```python
from build123d import *

# Parameters (mm, degrees)
SKETCH1_R               = 7.5
BOSS_EXTRUDE1_DEPTH     = 3
SKETCH3_R               = 2.5
BOSS_EXTRUDE3_DEPTH     = 15
FILLET1_R               = 1
SKETCH4_R               = 12.375
SKETCH4_R_2             = 2.375
CUT_EXTRUDE_THIN1_DEPTH = 0.5


with BuildPart() as part:
    # Sketch1 → Boss-Extrude1 (new body)
    with BuildSketch(Plane.XY):
        Circle(SKETCH1_R)
    extrude(amount=BOSS_EXTRUDE1_DEPTH)

    # Sketch3 → Boss-Extrude3 (add)
    with BuildSketch(Plane.XY.offset(3)):
        Circle(SKETCH3_R)
    extrude(amount=BOSS_EXTRUDE3_DEPTH)

    # Fillet1
    fillet1_edges = [part.edges().sort_by_distance(p)[0] for p in [
        (-7.5, 0, 0),
        (-2.5, 0, 18),
    ]]
    fillet(fillet1_edges, radius=FILLET1_R)

    # Sketch4 → Cut-Extrude-Thin1 (cut)
    with BuildSketch(Plane.XY.offset(15)):
        Circle(SKETCH4_R)
        Circle(SKETCH4_R_2, mode=Mode.SUBTRACT)
    extrude(amount=CUT_EXTRUDE_THIN1_DEPTH, mode=Mode.SUBTRACT)


solid = part.part
```
Model file for the job. Use its own axes, mm. Coordinates: 2 decimals unless noted, no trailing zeros. Loops run counter-clockwise (first coordinate to the right, second up) from the corner with the lowest first, then second, coordinate; pieces in that order, holes last. Notation, with made-up numbers: (-10, 26.5) - (2, 26.5) arc R21 ccw to (2, 52.5) - close; hole circle Ø9 at (19, 74.25). An arc over 180 degrees is marked (long way). Answer as a JSON object with one key per item and string values. Group by question number.
(1) Cut at C-C (z = 15.25). Give the cut face in (x, y) (3 decimals), then the cut area to 3 significant figures.
(2) Flat gauge pins, fed straight in: pin 1 (6 mm diameter, centred on x = 5.5, z = 4, fed in from -Y); pin 2 (8 mm diameter, centred on y = 6, z = 6, fed in from -X). Where does each tip first touch, or does it go through?
(3) Cut at A-A (y = 0). Give the cut face in (x, z) (3 decimals).
(4) Probe line 1 along Z through (x, y) = (-2.75, -4); line 2 along X through (y, z) = (2, 5.5); line 3 along Z through (x, y) = (0, -1.75). List the from-to ranges inside material, lowest first.
(5) Cut at D-D (z = 5.75). Give the cut face in (x, y).
(6) Two-plate mould, pull along Z, no slides. Class faces 1 (the face through (1.096, -2.107, 15.246)), 2 (the face through (0, 0, 18)), 3 (the face through (-7.493, 0.33, 1.986)), 4 (the face through (0, 0, 0)): released by +Z, released by -Z, zero draft, split by the parting line, or undercut.
Geometry says:
{
 "1": {"outline": "circle Ø4.75 at (0, 0)", "area": "17.7 mm^2"},
 "2": {"pin 1": "stops at y = -7.01", "pin 2": "stops at x = -6.71"},
 "3": {"outline": "(-7.5, 1) arc R1 ccw to (-6.5, 0) - (6.5, 0) arc R1 ccw to (7.5, 1) - (7.5, 3) - (2.5, 3) - (2.5, 15) - (2.375, 15) - (2.375, 15.5) - (2.5, 15.5) - (2.5, 17) arc R1 ccw to (1.5, 18) - (-1.5, 18) arc R1 ccw to (-2.5, 17) - (-2.5, 15.5) - (-2.375, 15.5) - (-2.375, 15) - (-2.5, 15) - (-2.5, 3) - (-7.5, 3) - close"},
 "4": {"line 1": "z = 0 to 3", "line 2": "x = -1.5 to 1.5", "line 3": "z = 0 to 17.97"},
 "5": {"outline": "circle Ø5 at (0, 0)"},
 "6": {"face 1": "undercut", "face 2": "released by +Z", "face 3": "zero draft", "face 4": "released by -Z"}
}
